Could you check a few things on this model? Use its own coordinates, in mm. Round coordinates to 2 decimals unless told otherwise and drop trailing zeros. Loops run counter-clockwise (first coordinate to the right, second up) from the corner with the lowest first, then second, coordinate; pieces in that order, holes last.
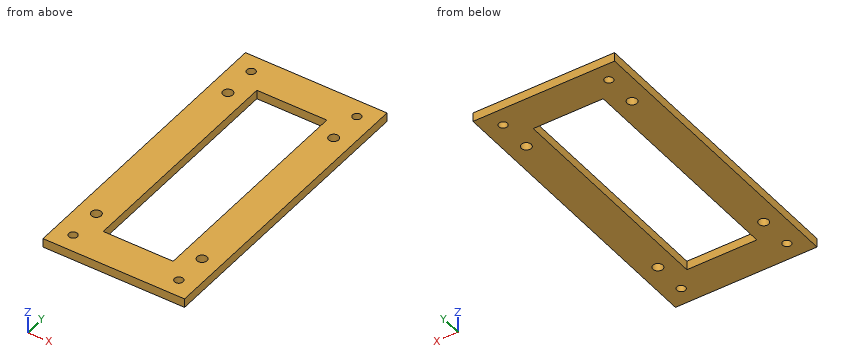
from build123d import *

# Parameters (mm, degrees)
SKETCH1_W           = 100.4
SKETCH1_H           = 210.8
SKETCH1_W_2         = 49.6
SKETCH1_H_2         = 160
BOSS_EXTRUDE1_DEPTH = 6.35
SKETCH2_R           = 3
CUT_EXTRUDE1_DEPTH  = 6.35
SKETCH3_R           = 3.5
CUT_EXTRUDE2_DEPTH  = 10


with BuildPart() as part:
    # Sketch1 → Boss-Extrude1 (new body)
    with BuildSketch(Plane.XY):
        with Locations((50.2, 105.4)):
            Rectangle(SKETCH1_W, SKETCH1_H)
        with Locations((50.2, 105.4)):
            Rectangle(SKETCH1_W_2, SKETCH1_H_2, mode=Mode.SUBTRACT)
    extrude(amount=BOSS_EXTRUDE1_DEPTH)

    # Sketch2 → Cut-Extrude1 (cut)
    with BuildSketch(Plane.XY.offset(6.35)):
        with Locations((12.70273435, 198.1)):
            Circle(SKETCH2_R)
        with Locations((87.69726565, 198.1)):
            Circle(SKETCH2_R)
        with Locations((87.69726565, 12.7)):
            Circle(SKETCH2_R)
        with Locations((12.70273435, 12.7)):
            Circle(SKETCH2_R)
    extrude(amount=-CUT_EXTRUDE1_DEPTH, mode=Mode.SUBTRACT)

    # Sketch3 → Cut-Extrude2 (cut)
    with BuildSketch(Plane.XY.offset(6.35)):
        with Locations((12.7, 173.9)):
            Circle(SKETCH3_R)
        with Locations((87.7, 173.9)):
            Circle(SKETCH3_R)
        with Locations((87.7, 36.9)):
            Circle(SKETCH3_R)
        with Locations((12.7, 36.9)):
            Circle(SKETCH3_R)
    extrude(amount=-CUT_EXTRUDE2_DEPTH, mode=Mode.SUBTRACT)


solid = part.part
Item 1: Will this pin go through, and if not, where does the flat tip stop? pin 1 (5 mm diameter, centred on x = 12.7, y = 198.1, fed in from +Z).
Results list:
pin 1: passes through
Item 2: If we section it at A-A, the plane y = 58: Please give me the cut outline in (x, z), then the cut area to 3 significant figures.
Results list:
outline: (0, 0) - (25.4, 0) - (25.4, 6.35) - (0, 6.35) - close; (75, 0) - (100.4, 0) - (100.4, 6.35) - (75, 6.35) - close
area: 323 mm2
Item 3: If I drill on line 1 along Y through (x, z) = (87.7, 4.25); line 2 along X through (y, z) = (198.1, 2.25); line 3 along Y through (x, z) = (74, 4), over which ranges is the centre line in solid material (lowest first)?
Results list:
line 1: y = 0 to 9.7, 15.7 to 33.4, 40.4 to 170.4, 177.4 to 195.1, 201.1 to 210.8
line 2: x = 0 to 9.7, 15.7 to 84.7, 90.7 to 100.4
line 3: y = 0 to 25.4, 185.4 to 210.8
Item 4: If we section it at C-C, the plane z = 2.25: Count the separate pieces of the cut face and the enclosed holes in it, then the cut area to 3 significant figures.
Results list:
separate pieces: 1
enclosed holes: 9
area: 13,000 mm2
Item 5: If we section it at D-D, the plane y = 173.9: Please give me the cut outline in (x, z).
Results list:
outline: (0, 0) - (9.2, 0) - (9.2, 6.35) - (0, 6.35) - close; (16.2, 0) - (25.4, 0) - (25.4, 6.35) - (16.2, 6.35) - close; (75, 0) - (84.2, 0) - (84.2, 6.35) - (75, 6.35) - close; (91.2, 0) - (100.4, 0) - (100.4, 6.35) - (91.2, 6.35) - close
Item 6: If we section it at B-B, the plane x = 68: Please give me the cut outline in (y, z), then the cut area to 3 significant figures.
Results list:
outline: (0, 0) - (25.4, 0) - (25.4, 6.35) - (0, 6.35) - close; (185.4, 0) - (210.8, 0) - (210.8, 6.35) - (185.4, 6.35) - close
area: 323 mm2
